Autodesk Inventor part; units mm, degrees
ref_plane "Work Plane1" through (-12.5, 10, 0) normal (0, 1, 0) x (1, 0, 0)
ref_plane "YZ Plane" through (0, 0, 0) normal (1, 0, 0) x (0, 1, 0)
ref_plane "XZ Plane" through (0, 0, 0) normal (0, 1, 0) x (-1, 0, 0)
sketch "Sketch1" plane through (0, 0, 0) normal (0, 0, 1) x (1, 0, 0)
  line L0 (-17.5, 0) -> (17.5, 0) construction
  line L1 (0, -17.5) -> (0, 17.5) construction
  line L2 (-12.5, -12.5) -> (12.5, -12.5)
  line L3 (12.5, -12.5) -> (12.5, 12.5)
  line L4 (12.5, 12.5) -> (-12.5, 12.5)
  line L5 (-12.5, 12.5) -> (-12.5, -12.5)
  line L6 (-12.5, -12.5) -> (12.5, 12.5) construction
  line L7 (12.5, -12.5) -> (-12.5, 12.5) construction
  point P0 (0, 0)
  dimension "d0" = 25
  dimension "d1" = 25
extrude "Extrusion1" add sketch "Sketch1" along normal blind 5
ref_plane "Work Plane1" through (-12.5, 10, 0) normal (0, 1, 0) x (1, 0, 0)
sketch "Sketch2" plane through (-12.5, 10, 0) normal (0, 1, 0) x (1, 0, 0)
  line L0 (25, 0) -> (0, 0) construction
  line L1 (0, 0) -> (0, -5) construction
  line L2 (25, -5) -> (0, -5) construction
  line L3 (25, 0) -> (25, -5) construction
  line L4 (12.5, 0) -> (12.5, -5) construction
  circle A0 centre (12.5, -35.334) radius 34.284
  line L5 (-3.4763, -5) -> (28.4763, -5)
  dimension "d5" = 68.568
  dimension "d6" = 30.334
extrude "Extrusion2" cut sketch "Sketch2" against normal blind 20
properties part number "00_cylindrical_lens_mould"
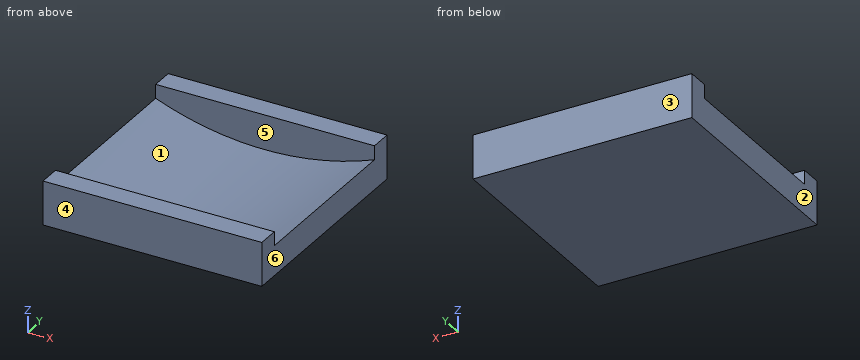
Design review of the part built by this model. Coordinates are the model's own, in mm. Face numbers are marked on the shaded views. A direction names the side the tool comes from. Give positions to 0.01 mm unless a question says otherwise; leave off trailing zeros. Order: outer loops, then holes, each group sorted by start corner. A loop starts at its lowest first (then second) coordinate and runs counter-clockwise, first axis right, second up. Notation, with made-up numbers: M 56,-8 L 88,-8 A23 cw 88,9 Z; hole C 53,81.25 d4. An arc over 180 degrees is marked long. One line per question, with ' | ' between items. Start each with the question number.
Q1. We need section D-D (x = 6.5). Write out the cut boundary in (y, z), plus the area to 3 significant figures.
Q2. For L1, parallel to Y at x = 0, z = 1.65; L2, parallel to Z at x = 0.5, y = 1; L3, parallel to Z at x = 11, y = 1, list the stretches that pass through material, from the lowest coordinate up. Write a range as [from, to].
Q3. We need section A-A (z = 4.65). Write out the cut boundary in (x, y).
Q4. We need section B-B (x = -4.75). Write out the cut boundary in (y, z).
Q5. For pin 1 Ø3 at (x, y) = (-9.5, -6) entering from -Z, flat-tipped, find the tip position at first contact; note if it passes through.
Q6. Machinability: for the marked faces 5 and 6, which of the approach directions +Z, -Z, +X, -X, +Y, -Y give a long, thin tool a straight path to every point of the face, cutting with its end or side? Answer none if there is none.
Q7. We need section C-C (y = -8). Write out the cut boundary in (x, z).
Q8. The part is to be moulded in two halves that separate along Y. For the marked faces 1, 2, 3 and 4, say which applies: +Y half, -Y half, draft (parallel to the pull), parting line (faces both ways), or undercut.
Returned:
1) outline: M -12.5,0 L 12.5,0 L 12.5,5 L 10,5 L 10,1.67 L -10,1.67 L -10,5 L -12.5,5 Z | area: 58.4 mm2
2) L1: [-12.5, -10], [10, 12.5] | L2: [0, 1.05] | L3: [0, 2.86]
3) outline: M -12.5,-12.5 L 12.5,-12.5 L 12.5,-10 L -12.5,-10 Z; M -12.5,10 L 12.5,10 L 12.5,12.5 L -12.5,12.5 Z
4) outline: M -12.5,0 L 12.5,0 L 12.5,5 L 10,5 L 10,1.38 L -10,1.38 L -10,5 L -12.5,5 Z
5) pin 1: z = 0
6) face 5: +Z | face 6: +Z, -Z, +X, +Y, -Y
7) outline: M -12.5,0 L 12.5,0 L 12.5,3.41 A34.28 cw -12.5,3.41 Z
8) face 1: undercut | face 2: draft | face 3: +Y half | face 4: -Y half
